from build123d import *

# Parameters (mm, degrees)
F0_W     = 100
F0_H     = 60
F1_DEPTH = 30
F2_W     = 90.000001
F2_H     = 50.000001
F3_DEPTH = 20
F4_R     = 10
F5_DEPTH = 5
F6_R     = 1


with BuildPart() as f1:
    # F0 (on Top) → F1 (new body)
    with BuildSketch(Plane.XY):
        with Locations((-5.040722, 46.412729)):
            Rectangle(F0_W, F0_H)
    extrude(amount=F1_DEPTH)

    # F2 (on face) → F3 (cut)
    with BuildSketch(Plane(origin=(0, 0, 0), x_dir=(1, 0, 0), z_dir=(0, 0, -1))):
        with Locations((-5.040722, -46.412729)):
            Rectangle(F2_W, F2_H)
    extrude(amount=-F3_DEPTH, mode=Mode.SUBTRACT)

    # F4 (on face) → F5 (join)
    with BuildSketch(Plane.XY.offset(30)):
        with Locations((-30.040722, 61.412729)):
            Circle(F4_R)
        with Locations((-30.040722, 31.412729)):
            Circle(F4_R)
        with Locations((19.959278, 61.412729)):
            Circle(F4_R)
        with Locations((19.959278, 31.412729)):
            Circle(F4_R)
    extrude(amount=F5_DEPTH)

    # F6
    f6_edges = [f1.edges().sort_by_distance(p)[0] for p in [
        (-40.040722, 61.412729, 35),
        (9.959278, 61.412729, 35),
        (9.959278, 31.412729, 35),
        (-40.040722, 31.412729, 35),
    ]]
    fillet(f6_edges, radius=F6_R)


solid = f1.part
Read the model definition and answer for the solid it produces. Units are mm, in the model's axes. A direction names the side the tool comes from. Give positions to 0.01 mm unless a question says otherwise; leave off trailing zeros. Write each loop counter-clockwise with the first axis right and the second up, starting at its lowest first coordinate (ties: lowest second). Pieces come first, ordered by that corner, then holes. Notation, with made-up numbers: (82, 81.25) -> (100, 81.25) arc R19 cw to (100, 90.25) -> close; hole circle Ø3 at (27, -12). An arc over 180 degrees is marked (long way). Answer as a JSON object with one key per item and string values. Group by question number.
1) Each of these flat-tipped pins is pushed along its axis until it touches: P1, Ø18, axis at x = -6, y = 42.5, coming from the +Z side; P2, Ø2, axis at x = -26, y = 64.5, coming from the -Z side. Where does it stop, or does it pass through?
2) Find section A-A (z = 13). Write down the section's boundary in (x, y).
3) Find section C-C (x = -9). Write down the section's boundary in (y, z).
4) The mould has two halves that part along Y. Classify faces 1 (the flat face through (-6, 76.413, 15)), 2 (the flat face through (-30, 32, 35)), 3 (the flat face through (-6, 46, 20)): +Y half, -Y half, draft (parallel to the pull), parting line (faces both ways), or undercut.
5) Find section B-B (y = 42.5). Write down the section's boundary in (x, z), and give its area (3 significant figures).
6) A tool of negligible diameter and unlimited length cuts with its end or side. For faces 4 (the cylindrical face through (-31.343, 71.328, 31.972)), 5 (the flat face through (20, 62, 35)), 6 (the flat face through (-6, 21.413, 10)), from which of +Z, -Z, +X, -X, +Y, -Y can it reach the whole face along a straight path? Write none if from no direction.
7) Consider L1, parallel to Y at x = -48.5, z = 14; L2, parallel to X at y = 67, z = 6.5; L3, parallel to Z at x = -33, y = 35.5. Determine where each line is inside the solid, lowest interval first. Write a range as from..to.
Values follow:
{
 "1": {"P1": "stops at z = 30", "P2": "stops at z = 20"},
 "2": {"outline": "(-55.04, 16.41) -> (44.96, 16.41) -> (44.96, 76.41) -> (-55.04, 76.41) -> close; hole (-50.04, 21.41) -> (39.96, 21.41) -> (39.96, 71.41) -> (-50.04, 71.41) -> close"},
 "3": {"outline": "(16.41, 0) -> (21.41, 0) -> (21.41, 20) -> (71.41, 20) -> (71.41, 0) -> (76.41, 0) -> (76.41, 30) -> (16.41, 30) -> close"},
 "4": {"face 1": "+Y half", "face 2": "draft", "face 3": "undercut"},
 "5": {"outline": "(-55.04, 0) -> (-50.04, 0) -> (-50.04, 20) -> (39.96, 20) -> (39.96, 0) -> (44.96, 0) -> (44.96, 30) -> (-55.04, 30) -> close", "area": "1,200 mm2"},
 "6": {"face 4": "+Z", "face 5": "+Z, +X, -X, +Y, -Y", "face 6": "-Z"},
 "7": {"L1": "y = 16.41..21.41, 71.41..76.41", "L2": "x = -55.04..-50.04, 39.96..44.96", "L3": "z = 20..35"}
}
